Here's the drawing with two shaded views (mm, measured from the low corner). I have some questions. A direction names the side the tool comes from. Give positions to 0.01 mm unless a question says otherwise; leave off trailing zeros. Loops run counter-clockwise (first coordinate to the right, second up) from the corner with the lowest first, then second, coordinate; pieces in that order, holes last. Notation, with made-up numbers: M -19,-26.5 L 18,-26.5 A20 cw 18,-11.5 Z; hole C 33,4 d10. An arc over 180 degrees is marked long. Use a Markdown table: item, result. Add a question column.
1) Suppose I cut it at D-D on x = 13.5. List the corners of the cut face in (y, z) for me, and give its area (3 significant figures).
2) Suppose I cut it at C-C on y = 6.75. List the corners of the cut face in (x, z) for me, and give its area (3 significant figures).
3) Suppose I cut it at B-B on x = 28.3. List the corners of the cut face in (y, z) for me, and give its area (3 significant figures).
4) If I drill on line 1 along X through (y, z) = (23.65, 28.3); line 2 along X through (y, z) = (9.25, 28), over which ranges is the centre line in solid material (lowest first)? Write a range as [from, to].
5) Which directions (+Z, -Z, +X, -X, +Y, -Y) give clear straight access to the entire face, cutting with the end or side of a thin tool? Please do the marked faces 5, 6 and 7.
6) Will these pins go through, and if not, where does the flat tip stop? pin 1 Ø1 at (x, y) = (22.5, 3) entering from -Z; pin 2 Ø5 at (y, z) = (4, 39.5) entering from -X; pin 3 Ø12 at (x, z) = (27, 27) entering from +Y; pin 4 Ø9 at (x, z) = (28.3, 28.3) entering from -Y.
7) Suppose I cut it at A-A on z = 28.3. List the corners of the cut face in (x, y) for me, and give its area (3 significant figures).
8) We'd pull the mould along Z, two halves only. Please class the marked faces 1, 2, 3 and 4: +Z half, -Z half, draft (parallel to the pull), parting line (faces both ways), or undercut.
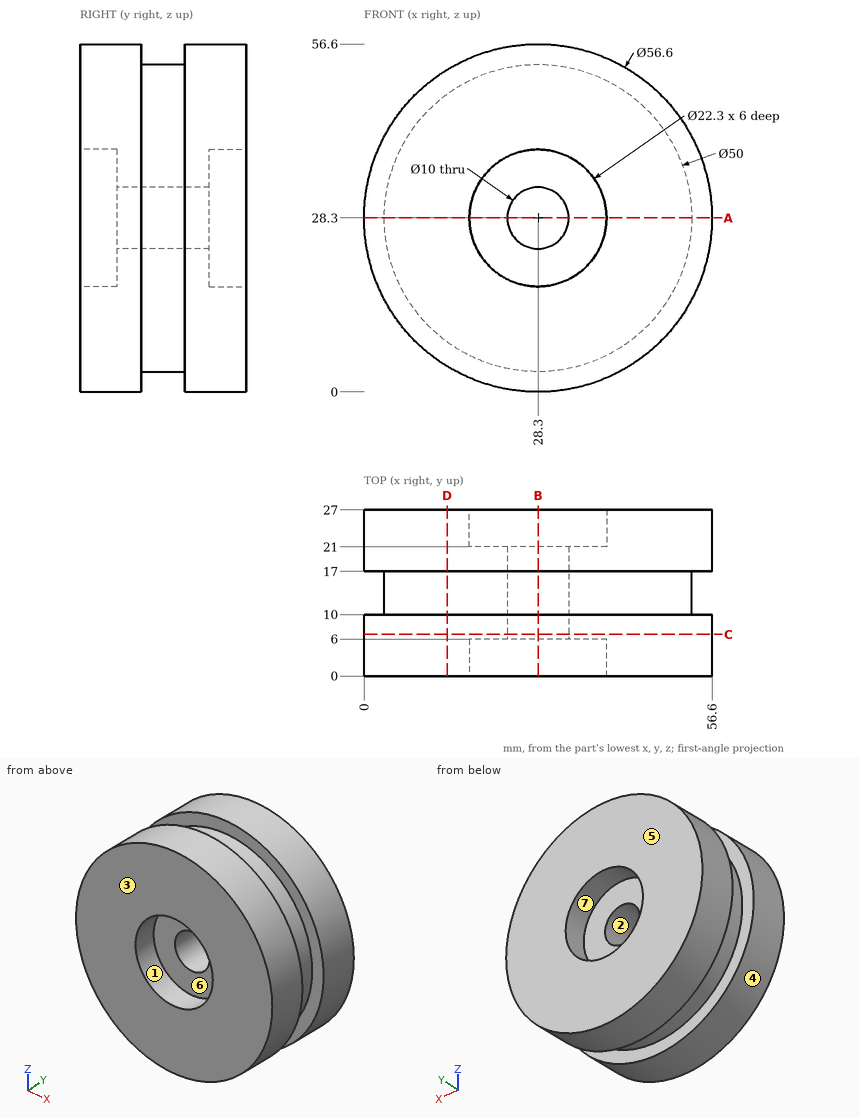
Answer block:
| question | item | result |
|---|---|---|
| 1 | outline | M 0,4.18 L 10,4.18 L 10,8.15 L 17,8.15 L 17,4.18 L 27,4.18 L 27,52.42 L 17,52.42 L 17,48.45 L 10,48.45 L 10,52.42 L 0,52.42 Z |
| 1 | area | 1,250 mm^2 |
| 2 | outline | C 28.3,28.3 d56.6; hole C 28.3,28.3 d10 |
| 2 | area | 2,440 mm^2 |
| 3 | outline | M 0,0 L 10,0 L 10,3.3 L 17,3.3 L 17,0 L 27,0 L 27,17.15 L 21,17.15 L 21,23.3 L 6,23.3 L 6,17.15 L 0,17.15 Z; M 0,39.45 L 6,39.45 L 6,33.3 L 21,33.3 L 21,39.45 L 27,39.45 L 27,56.6 L 17,56.6 L 17,53.3 L 10,53.3 L 10,56.6 L 0,56.6 Z |
| 3 | area | 1,060 mm^2 |
| 4 | line 1 | x = [0, 17.15], [39.45, 56.6] |
| 4 | line 2 | x = [0, 23.31], [33.29, 56.6] |
| 5 | face 5 | +Z, -Z, +X, -X, +Y |
| 5 | face 6 | -Y |
| 5 | face 7 | +Y |
| 6 | pin 1 | stops at z = 0.5 |
| 6 | pin 2 | stops at x = 1.37 |
| 6 | pin 3 | stops at y = 21 |
| 6 | pin 4 | passes through |
| 7 | outline | M 0,0 L 17.15,0 L 17.15,6 L 23.3,6 L 23.3,21 L 17.15,21 L 17.15,27 L 0,27 L 0,17 L 3.3,17 L 3.3,10 L 0,10 Z; M 33.3,6 L 39.45,6 L 39.45,0 L 56.6,0 L 56.6,10 L 53.3,10 L 53.3,17 L 56.6,17 L 56.6,27 L 39.45,27 L 39.45,21 L 33.3,21 Z |
| 7 | area | 1,060 mm^2 |
| 8 | face 1 | undercut |
| 8 | face 2 | undercut |
| 8 | face 3 | draft |
| 8 | face 4 | parting line |
